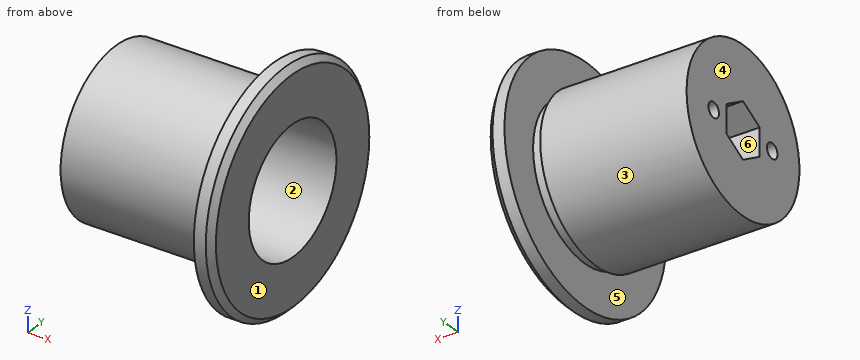
from build123d import *

# Parameters (mm, degrees)
CUT_EXTRUDE_1_DEPTH = 30.4
CHAMFER_1_SIZE      = 1
SKETCH_3_R          = 1.25
CUT_EXTRUDE_2_DEPTH = 30.4


with BuildPart() as part:
    # 草图1 → 旋转1 (revolve)
    with BuildSketch(Plane.XY):
        Polygon((29.4, 19.35), (29.4, 10.5), (8, 10.5), (8, 0), (0, 0), (0, 13.5), (24.5, 13.5), (24.5, 12.5), (26.4, 12.5), (26.4, 19.35), align=None)
    revolve(axis=Axis((0, 0, 0), (1, 0, 0)))

    # 草图2 → 切除-拉伸1 (cut, through all)
    with BuildSketch(Plane(origin=(29.4, 0, 0), x_dir=(0, 0, -1), z_dir=(1, 0, 0))):
        Polygon((-2.309401077, 4), (-4.618802154, 0), (-2.309401077, -4), (2.309401077, -4), (4.618802154, 0), (2.309401077, 4), align=None)
    extrude(amount=-CUT_EXTRUDE_1_DEPTH, mode=Mode.SUBTRACT)

    # 倒角1
    chamfer_1_edges = [part.edges().sort_by_distance(p)[0] for p in [
        (29.4, -19.35, 0),
    ]]
    chamfer(chamfer_1_edges, length=CHAMFER_1_SIZE)

    # 草图3 → 切除-拉伸2 (cut, through all)
    with BuildSketch(Plane(origin=(29.4, 0, 0), x_dir=(0, 0, -1), z_dir=(1, 0, 0))):
        with Locations((0, 7)):
            Circle(SKETCH_3_R)
        with Locations((0, -7)):
            Circle(SKETCH_3_R)
    extrude(amount=-CUT_EXTRUDE_2_DEPTH, mode=Mode.SUBTRACT)


solid = part.part
Read the model definition and answer for the solid it produces. Units are mm, in the model's axes. Face numbers are marked on the shaded views. A direction names the side the tool comes from. Round coordinates to 2 decimals unless told otherwise and drop trailing zeros. Order: outer loops, then holes, each group sorted by start corner. A loop starts at its lowest first (then second) coordinate and runs counter-clockwise, first axis right, second up. Notation, with made-up numbers: (3, 75) - (52, 75) arc R14 ccw to (52, 80) - close; hole circle Ø8 at (3.5, -39.5). An arc over 180 degrees is marked (long way). Use one line per item in the form item = value. Start each with the question number.
(1) For the marked faces 4, 5 and 6, determine the directions among +Z, -Z, +X, -X, +Y, -Y from which every point of the face is accessible in a straight line to the end or side of a thin tool.
(2) The part is cut by section A-A (z = 0). Count the separate pieces of the cut face and the enclosed holes in it, then the cut area to 3 significant figures.
(3) The part is cut by section B-B (x = 15.5). Give the vertices of the cut face in (y, z).
(4) Flat-ended cylindrical pins translate along their axes: pin 1 Ø1 at (y, z) = (-8, 15) entering from -X; pin 2 Ø12 at (x, y) = (10.5, -4) entering from -Z; pin 3 Ø1.4 at (x, z) = (6, -1) entering from -Y. Find the tip coordinate at first contact, or state that the pin passes through.
(5) Determine the mould class of the marked faces 1, 2 and 3 for opening direction Y: +Y half, -Y half, draft (parallel to the pull), parting line (faces both ways), or undercut.
(6) Find the intervals of material crossed by line 1 along X through (y, z) = (-13, -1.5); line 2 along X through (y, z) = (8, -14); line 3 along Z through (x, y) = (13.25, 0), in increasing order. Write a range as from..to.
Checked values:
q1.face_4 = +Z, -Z, -X, +Y, -Y
q1.face_5 = none
q1.face_6 = +X, -X
q2.separate_pieces = 4
q2.enclosed_holes = 0
q2.area = 271 mm^2
q3.outline = circle Ø27 at (0, 0); hole circle Ø21 at (0, 0)
q4.pin_1 = 26.4
q4.pin_2 = -13.5
q4.pin_3 = -13.5
q5.face_1 = draft
q5.face_2 = undercut
q5.face_3 = parting line
q6.line_1 = 0..24.5, 26.4..29.4
q6.line_2 = 26.4..29.4
q6.line_3 = -13.5..-10.5, 10.5..13.5
